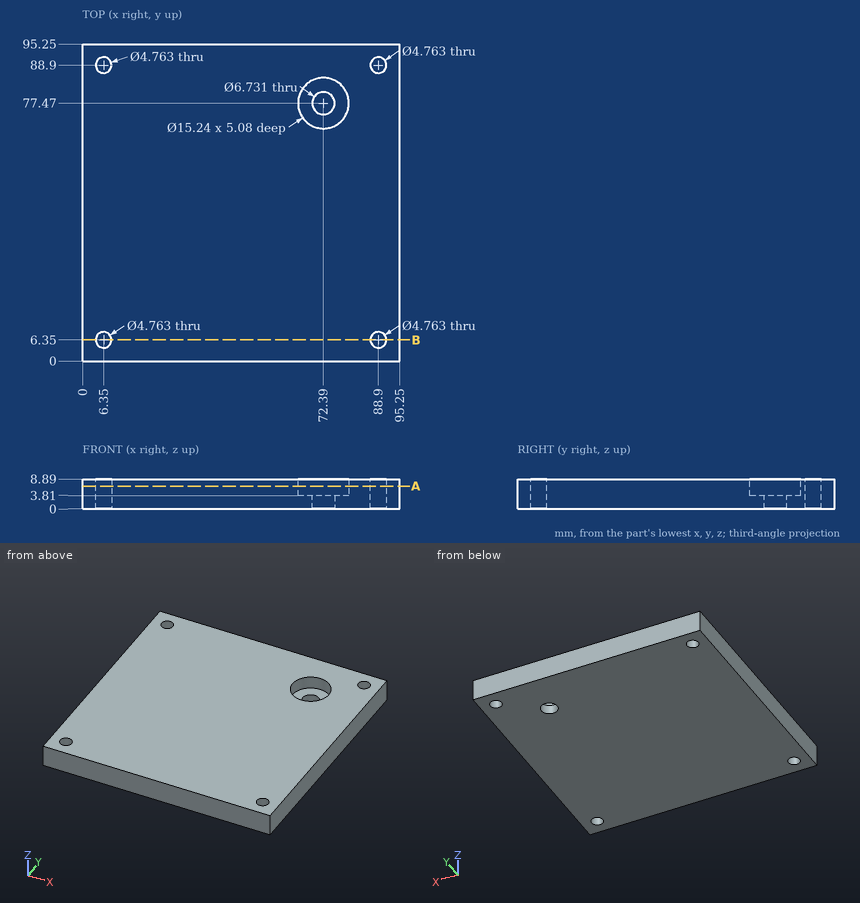
Answer from the drawing. Dimensions are ordinates in mm from the lowest x, y and z of the part. Coordinates: 2 decimals unless noted, no trailing zeros. Write each loop counter-clockwise with the first axis right and the second up, starting at its lowest first coordinate (ties: lowest second). Pieces come first, ordered by that corner, then holes. Notation, with made-up numbers: M 51.5,72.25 L 64.5,72.25 A33 ccw 64.5,100.25 Z; hole C -35,49 d10. An arc over 180 degrees is marked long. Use a Markdown table: item, result.
Q1. This flat-tipped pin is pushed along its axis until it touches: pin 1 Ø4.5 at (x, y) = (88.9, 88.9) entering from +Z. Where does it stop, or does it pass through?
Answer block:
| item | result |
|---|---|
| pin 1 | passes through |
Q2. The part is cut by section A-A, the plane z = 6.75. Write down the section's boundary in (x, y), then the cut area to 3 significant figures.
Answer block:
| item | result |
|---|---|
| outline | M 0,0 L 95.25,0 L 95.25,95.25 L 0,95.25 Z; hole C 6.35,6.35 d4.76; hole C 6.35,88.9 d4.76; hole C 72.39,77.47 d15.24; hole C 88.9,6.35 d4.76; hole C 88.9,88.9 d4.76 |
| area | 8,820 mm2 |
Q3. The part is cut by section B-B, the plane y = 6.35. Write down the section's boundary in (x, z), then the cut area to 3 significant figures.
Answer block:
| item | result |
|---|---|
| outline | M 0,0 L 3.97,0 L 3.97,8.89 L 0,8.89 Z; M 8.73,0 L 86.52,0 L 86.52,8.89 L 8.73,8.89 Z; M 91.28,0 L 95.25,0 L 95.25,8.89 L 91.28,8.89 Z |
| area | 762 mm2 |
Q4. Straight lines are drawn through the part: L1, parallel to Y at x = 6.35, z = 5; L2, parallel to Y at x = 74, z = 7.25. For each, find the intervals that lie inside material, in ascending order. Write a range as [from, to].
Answer block:
| item | result |
|---|---|
| L1 | y = [0, 3.97], [8.73, 86.52], [91.28, 95.25] |
| L2 | y = [0, 70.02], [84.92, 95.25] |
